Answer from the drawing. Dimensions are ordinates in mm from the lowest x, y and z of the part. A direction names the side the tool comes from. Give positions to 0.01 mm unless a question says otherwise; leave off trailing zeros. Order: outer loops, then holes, each group sorted by start corner. A loop starts at its lowest first (then second) coordinate and runs counter-clockwise, first axis right, second up.
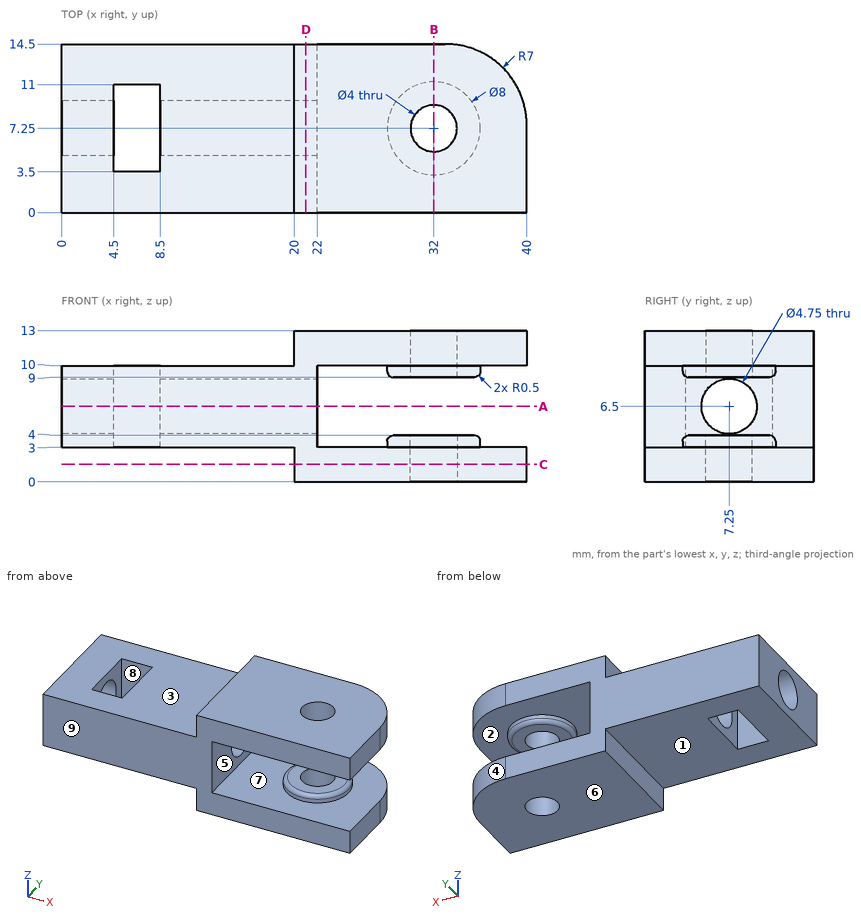
1) The part is cut by section B-B on x = 32. Determine the outline of the cut face in (y, z), and give its area (3 significant figures).
Final values:
outline: (0, 0) - (5.25, 0) - (5.25, 4) - (3.75, 4) arc R0.5 ccw to (3.25, 3.5) - (3.25, 3) - (0, 3) - close; (0, 10) - (3.25, 10) - (3.25, 9.5) arc R0.5 ccw to (3.75, 9) - (5.25, 9) - (5.25, 13) - (0, 13) - close; (9.25, 0) - (14.5, 0) - (14.5, 3) - (11.25, 3) - (11.25, 3.5) arc R0.5 ccw to (10.75, 4) - (9.25, 4) - close; (9.25, 9) - (10.75, 9) arc R0.5 ccw to (11.25, 9.5) - (11.25, 10) - (14.5, 10) - (14.5, 13) - (9.25, 13) - close
area: 70.8 mm2
2) The part is cut by section D-D on x = 21. Determine the outline of the cut face in (y, z) (3 decimals), and give its area (3 significant figures).
Final values:
outline: (0, 0) - (14.5, 0) - (14.5, 13) - (0, 13) - close; hole circle Ø4.75 at (7.25, 6.5)
area: 171 mm2
3) Consider L1, parallel to Y at x = 7.5, z = 7; L2, parallel to Z at x = 30.5, y = 13.75; L3, parallel to X at y = 10.25, z = 7. Determine where each line is inside the solid, lowest interval first.
Final values:
L1: y = 0 to 3.5, 11 to 14.5
L2: z = 0 to 3, 10 to 13
L3: x = 0 to 4.5, 8.5 to 22
4) The part is cut by section A-A on z = 6.5. Determine the outline of the cut face in (x, y) (3 decimals), and give its area (4 significant figures).
Final values:
outline: (0, 0) - (22, 0) - (22, 4.875) - (8.5, 4.875) - (8.5, 3.5) - (4.5, 3.5) - (4.5, 4.875) - (0, 4.875) - close; (0, 9.625) - (4.5, 9.625) - (4.5, 11) - (8.5, 11) - (8.5, 9.625) - (22, 9.625) - (22, 14.5) - (0, 14.5) - close
area: 203.5 mm2
5) The part is cut by section C-C on z = 1.5. Determine the outline of the cut face in (x, y).
Final values:
outline: (20, 0) - (40, 0) - (40, 7.5) arc R7 ccw to (33, 14.5) - (20, 14.5) - close; hole circle Ø4 at (32, 7.25)
6) Given pin 1 (8 mm diameter, centred on x = 6.5, y = 6, fed in from +Z); pin 2 (1.5 mm diameter, centred on y = 7.5, z = 11.5, fed in from -X), each flat-ended and moving along its own axis, determine where each tip first touches the part or whether it passes through.
Final values:
pin 1: stops at z = 10
pin 2: stops at x = 20
7) For a pull along Z with two mould halves and no side action, classify the marked faces 1, 2, 3 and 4 as released by +Z, released by -Z, zero draft, split by the parting line, or undercut.
Final values:
face 1: released by -Z
face 2: undercut
face 3: released by +Z
face 4: zero draft
8) A tool of negligible diameter and unlimited length cuts with its end or side. For the marked faces 5, 6, 7, 8 and 9, from which of +Z, -Z, +X, -X, +Y, -Y can it reach the whole face along a straight path? Write none if from no direction.
Final values:
face 5: +Y, -Y
face 6: -Z, +X, -X, +Y, -Y
face 7: none
face 8: +Z, -Z
face 9: +Z, -Z, +X, -X, -Y
